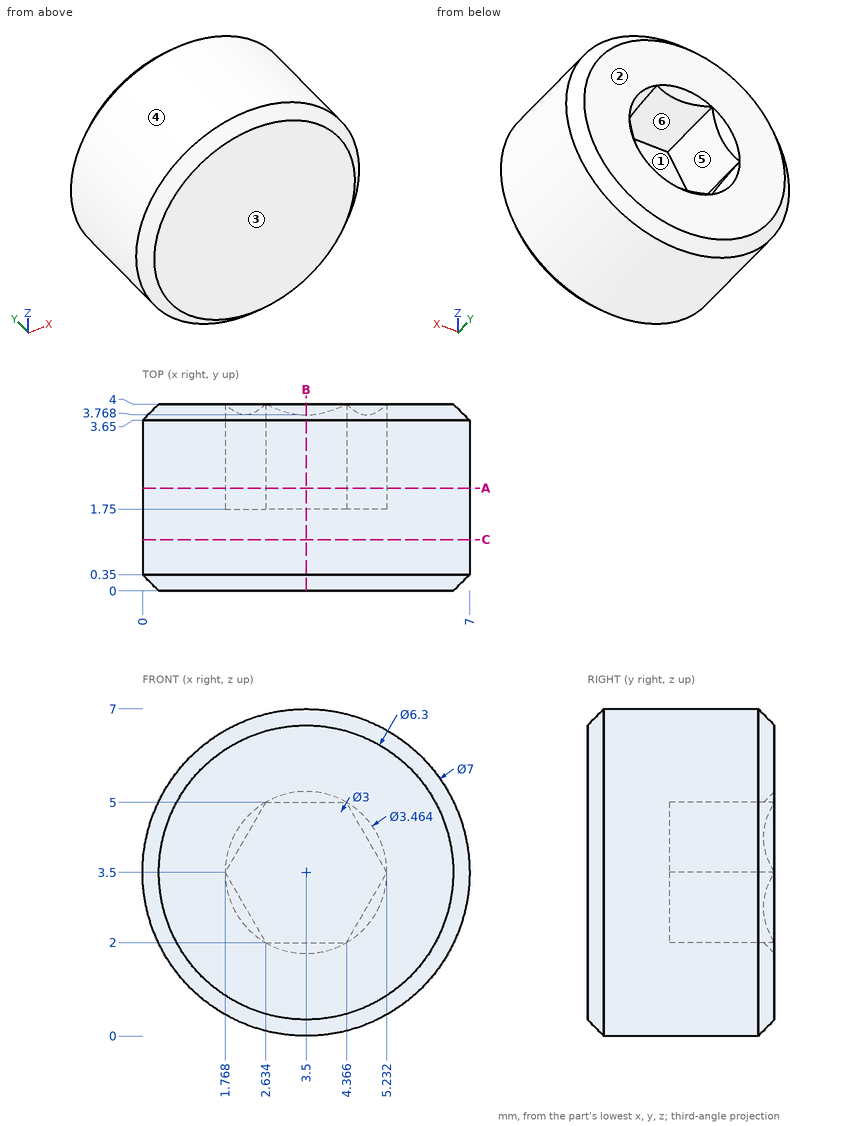
Input: dimensioned drawing with shaded views. Units: mm. Origin: part minimum x, y, z. A direction names the side the tool comes from. Coordinates: 2 decimals unless noted, no trailing zeros. Order: outer loops, then holes, each group sorted by start corner. A loop starts at its lowest first (then second) coordinate and runs counter-clockwise, first axis right, second up.
1. Cut plane B-B, the plane x = 3.5. Return loops of the section in (y, z).
Checked values:
outline: (0, 0.35) - (0.35, 0) - (3.65, 0) - (4, 0.35) - (4, 1.77) - (3.77, 2) - (1.75, 2) - (1.75, 5) - (3.77, 5) - (4, 5.23) - (4, 6.65) - (3.65, 7) - (0.35, 7) - (0, 6.65) - close
2. Cut plane A-A, the plane y = 2.2. Return loops of the section in (x, z), plus the area to 3 significant figures.
Checked values:
outline: circle Ø7 at (3.5, 3.5); hole (1.77, 3.5) - (2.63, 2) - (4.37, 2) - (5.23, 3.5) - (4.37, 5) - (2.63, 5) - close
area: 30.7 mm2
3. Contact query for flat-ended pins moving along their axis: P1, Ø2.5, axis at x = 4, z = 3, coming from the +Y side; P2, Ø0.5, axis at x = 4, y = 3, coming from the +Z side; P3, Ø2, axis at y = 1, z = 1, coming from the -X side. Output: stop coordinate, or through.
Checked values:
P1: stops at y = 4
P2: stops at z = 6.99
P3: stops at x = 0.34
4. Cut plane C-C, the plane y = 1.1. Return loops of the section in (x, z).
Checked values:
outline: circle Ø7 at (3.5, 3.5)
5. Draft query along Z for the marked faces 3, 4, 5 and 6. Return one class per face: +Z half, -Z half, draft (parallel to the pull), parting line (faces both ways), or undercut.
Checked values:
face 3: draft
face 4: parting line
face 5: undercut
face 6: undercut
6. Ray query, line 1 along X through (y, z) = (2.55, 3); line 2 along Z through (x, y) = (5, 2.4); line 3 along Y through (x, z) = (4, 2.25). Return the intervals inside material, ascending.
Checked values:
line 1: x = 0.04 to 2.06, 4.94 to 6.96
line 2: z = 0.34 to 3.1, 3.9 to 6.66
line 3: y = 0 to 1.75
7. Access query for the marked faces 1 and 2. Directions: +Z, -Z, +X, -X, +Y, -Y. A direction counts if a zero-diameter tool reaches every point of the face in a straight line with its end or side. Return the directions, or none.
Checked values:
face 1: +Y
face 2: +Z, -Z, +X, -X, +Y
